For this review, take the finished solid that the model builds, in its own axes (mm). Give positions to 0.01 mm unless a question says otherwise; leave off trailing zeros. Order: outer loops, then holes, each group sorted by start corner. A loop starts at its lowest first (then second) coordinate and runs counter-clockwise, first axis right, second up. Notation, with made-up numbers: (1.5, 29) -> (60.5, 29) arc R23 ccw to (60.5, 63) -> close; hole circle Ø2 at (66.5, -24). An arc over 180 degrees is marked (long way). Return JSON: item names as keys, results as strings. Group by question number.
1) Add section C-C (z = 29). Give the boundary of the cut face in (x, y), then the cut area to 3 significant figures.
2) Insertion check: P1, Ø16, axis at x = -38, y = 1.5, coming from the +Z side. The pin has a flat end and moves straight along its axis. Give the tip position at first contact, or say it passes through.
3) Add section D-D (y = 19). Give the boundary of the cut face in (x, z), then the cut area to 3 significant figures.
4) To check wall thickness, follow line 1 along Y through (x, z) = (0, 22); line 2 along Z through (x, y) = (58, 23); line 3 along Y through (x, z) = (7, 53). State the ranges of each line that lie inside material, in increasing order.
5) Add section B-B (y = 0). Give the boundary of the cut face in (x, z), then the cut area to 3 significant figures.
6) The part is to be moulded in two halves that separate along X. For faces 1 (the face through (30, 0, 67)), 2 (the face through (68, 0, 59)), 3 (the face through (-50, 0, 53)), 4 (the face through (-40, 0, 50)), say which applies: released by +X, released by -X, zero draft, split by the parting line, or undercut.
7) Add section A-A (x = 0). Give the boundary of the cut face in (y, z), then the cut area to 3 significant figures.
from build123d import *

# Parameters (mm, degrees)
F0_W     = 140
F0_H     = 60
F1_DEPTH = 60
F3_R     = 10
F5_DEPTH = 10
F4_R     = 10
F6_DEPTH = 96.3
F7_R     = 5
F2_R     = 10
F8_DEPTH = 10
F9_R     = 5


with BuildPart() as f1:
    # F0 (on Top) → F1 (new body)
    with BuildSketch(Plane.XY):
        Rectangle(F0_W, F0_H)
    extrude(amount=F1_DEPTH)

    # F3 (on face) → F5 (join)
    with BuildSketch(Plane.XY.offset(60)):
        with Locations((40, 0)):
            Circle(F3_R)
    extrude(amount=F5_DEPTH)

    # F4 (on face) → F6 (cut)
    with BuildSketch(Plane.XY.offset(60)):
        Circle(F4_R)
    extrude(amount=-F6_DEPTH, mode=Mode.SUBTRACT)

    # F7
    f7_edges = [f1.edges().sort_by_distance(p)[0] for p in [
        (0, -30, 0),
        (-70, 0, 0),
        (70, 0, 0),
        (0, 30, 0),
        (-10, 0, 0),
    ]]
    fillet(f7_edges, radius=F7_R)

    # F2 (on face) → F8 (cut)
    with BuildSketch(Plane.XY.offset(60)):
        with Locations((-40, 0)):
            Circle(F2_R)
    extrude(amount=-F8_DEPTH, mode=Mode.SUBTRACT)

    # F9
    f9_edges = [f1.edges().sort_by_distance(p)[0] for p in [
        (0, -30, 60),
        (-70, 0, 60),
        (70, 0, 60),
        (0, 30, 60),
        (-50, 0, 60),
        (-10, 0, 60),
        (30, 0, 60),
    ]]
    fillet(f9_edges, radius=F9_R)


solid = f1.part
Evaluation:
{
 "1": {"outline": "(-70, -30) -> (70, -30) -> (70, 30) -> (-70, 30) -> close; hole circle Ø20 at (0, 0)", "area": "8,090 mm^2"},
 "2": {"P1": "z = 57.18"},
 "3": {"outline": "(-70, 5) arc R5 ccw to (-65, 0) -> (65, 0) arc R5 ccw to (70, 5) -> (70, 55) arc R5 ccw to (65, 60) -> (-65, 60) arc R5 ccw to (-70, 55) -> close", "area": "8,380 mm^2"},
 "4": {"line 1": "-30 to -10, 10 to 30", "line 2": "0 to 60", "line 3": "-30 to -7.14, 7.14 to 30"},
 "5": {"outline": "(-70, 5) arc R5 ccw to (-65, 0) -> (-15, 0) arc R5 ccw to (-10, 5) -> (-10, 55) arc R5 ccw to (-15, 60) -> (-25, 60) arc R5 ccw to (-30, 55) -> (-30, 50) -> (-50, 50) -> (-50, 55) arc R5 ccw to (-55, 60) -> (-65, 60) arc R5 ccw to (-70, 55) -> close; (10, 5) arc R5 ccw to (15, 0) -> (65, 0) arc R5 ccw to (70, 5) -> (70, 55) arc R5 ccw to (65, 60) -> (55, 60) arc R5 cw to (50, 65) -> (50, 70) -> (30, 70) -> (30, 65) arc R5 cw to (25, 60) -> (15, 60) arc R5 ccw to (10, 55) -> close", "area": "7,160 mm^2"},
 "6": {"face 1": "split by the parting line", "face 2": "released by +X", "face 3": "undercut", "face 4": "undercut"},
 "7": {"outline": "(-30, 5) arc R5 ccw to (-25, 0) -> (-15, 0) arc R5 ccw to (-10, 5) -> (-10, 55) arc R5 ccw to (-15, 60) -> (-25, 60) arc R5 ccw to (-30, 55) -> close; (10, 5) arc R5 ccw to (15, 0) -> (25, 0) arc R5 ccw to (30, 5) -> (30, 55) arc R5 ccw to (25, 60) -> (15, 60) arc R5 ccw to (10, 55) -> close", "area": "2,360 mm^2"}
}
